from build123d import *

# Parameters (mm, degrees)
PAD_DEPTH       = 9
POCKET_DEPTH    = 6
SKETCH002_W     = 26.5
SKETCH002_H     = 35
POCKET001_DEPTH = 6
SKETCH003_W     = 192.75
SKETCH003_H     = 5.95
PAD001_DEPTH    = 3
SKETCH004_R     = 0.85
POCKET002_DEPTH = 541.411993
SKETCH005_W     = 26.5
SKETCH005_H     = 7.75
PAD002_DEPTH    = 3


with BuildPart() as part:
    # Sketch → Pad (new body)
    with BuildSketch(Plane.XY):
        with BuildLine():
            ThreePointArc((-92.5, 35), (-127.5, 0), (-92.5, -35))
            Line((-92.5, -35), (92.5, -35))
            ThreePointArc((92.5, -35), (127.5, 0), (92.5, 35))
            Line((-92.5, 35), (92.5, 35))
        make_face()
    extrude(amount=PAD_DEPTH)

    # Sketch001 (on Face6 of Pad) → Pocket (cut)
    with BuildSketch(Plane.XY.offset(9)):
        with BuildLine():
            ThreePointArc((-97.5, 6), (-103.5, 0), (-97.5, -6))
            Line((-97.5, -6), (97.5, -6))
            ThreePointArc((97.5, -6), (103.5, 0), (97.5, 6))
            Line((-97.5, 6), (97.5, 6))
        make_face()
    extrude(amount=-POCKET_DEPTH, mode=Mode.SUBTRACT)

    # Sketch002 (on Face5 of Pocket) → Pocket001 (cut)
    with BuildSketch(Plane.XY.offset(9)):
        with Locations((0, -17.5)):
            Rectangle(SKETCH002_W, SKETCH002_H)
    extrude(amount=-POCKET001_DEPTH, mode=Mode.SUBTRACT)

    # Sketch003 (on Face5 of Pocket001) → Pad001 (join)
    with BuildSketch(Plane.XY.offset(9)):
        with BuildLine():
            ThreePointArc((-92.5, 35), (-127.5, 0), (-92.5, -35))
            Line((-92.5, -35), (92.5, -35))
            ThreePointArc((92.5, -35), (127.5, 0), (92.5, 35))
            Line((-92.5, 35), (92.5, 35))
        make_face()
        Rectangle(SKETCH003_W, SKETCH003_H, mode=Mode.SUBTRACT)
    extrude(amount=PAD001_DEPTH)

    # Sketch004 (on Face12 of Pad001) → Pocket002 (cut, through all)
    with BuildSketch(Plane.XY.offset(12)):
        with Locations((-80, -8)):
            Circle(SKETCH004_R)
        with Locations((-63, -8)):
            Circle(SKETCH004_R)
        with Locations((-63, 8)):
            Circle(SKETCH004_R)
        with Locations((-80, 8)):
            Circle(SKETCH004_R)
    pocket002 = extrude(amount=-POCKET002_DEPTH, mode=Mode.SUBTRACT)

    # Sketch005 (on Face10 of Pocket002) → Pad002 (join)
    with BuildSketch(Plane.XY.offset(3)):
        with Locations((0, -37.125)):
            Rectangle(SKETCH005_W, SKETCH005_H)
    extrude(amount=PAD002_DEPTH)

    # Mirrored: Pocket002 across Sketch004 V_Axis
    add(pocket002.mirror(Plane(origin=(0, 0, 12), x_dir=(0, 0, 1), z_dir=(1, 0, 0))), mode=Mode.SUBTRACT)


solid = part.part
CAD build for the part. Positions are in the model's coordinates, mm. A direction names the side the tool comes from. Round coordinates to 2 decimals unless told otherwise and drop trailing zeros. Write each loop counter-clockwise with the first axis right and the second up, starting at its lowest first coordinate (ties: lowest second). Pieces come first, ordered by that corner, then holes. Notation, with made-up numbers: (65.5, -27) -> (107.5, -27) arc R35 ccw to (107.5, 8) -> close; hole circle Ø8 at (42.5, 30.5). An arc over 180 degrees is marked (long way). Answer as a JSON object with one key per item and string values.
(1) Band-saw the part on B-B, the plane y = -15. List the corners of the cut face in (x, z), then the cut area to 3 significant figures.
Reported:
{"outline": "(-124.12, 0) -> (124.12, 0) -> (124.12, 12) -> (-124.12, 12) -> close; hole (-13.25, 3) -> (13.25, 3) -> (13.25, 9) -> (-13.25, 9) -> close", "area": "2,820 mm^2"}
(2) Which spindle directions (+Z, -Z, +X, -X, +Y, -Y) get a long thin tool onto all of the face, cutting with end or side? Do faces 1 (the face through (-13.25, -21, 6)), 2 (the face through (0, -38, 3)), 3 (the face through (0, -37, 6)). Say none if no direction does.
Reported:
{"face 1": "none", "face 2": "-Z, +X, -X, -Y", "face 3": "-Y"}
(3) Pin check, flat tips, straight feed: P1, Ø1, axis at y = -32, z = 5, coming from the -X side; P2, Ø3.5, axis at y = -38, z = 4, coming from the +X side; P3, Ø4, axis at x = 91.5, z = 6, coming from the -Y side. Stop position of each tip, or through.
Reported:
{"P1": "stops at x = -107.76", "P2": "stops at x = 13.25", "P3": "stops at y = -35"}
(4) Band-saw the part on D-D, the plane y = 21.5. List the corners of the cut face in (x, z).
Reported:
{"outline": "(-120.12, 0) -> (120.12, 0) -> (120.12, 12) -> (-120.12, 12) -> close"}
(5) Probe probe 1 along Y at (x, z) = (-63, 3.5); probe 2 along Y at (x, z) = (63, 2.5); probe 3 along Y at (x, z) = (52, 4.5). List the from-to ranges inside material, lowest first. Write a range as [from, to].
Reported:
{"probe 1": "y = [-35, -8.85], [-7.15, -6], [6, 7.15], [8.85, 35]", "probe 2": "y = [-35, -8.85], [-7.15, 7.15], [8.85, 35]", "probe 3": "y = [-35, -6], [6, 35]"}
(6) Band-saw the part on C-C, the plane y = -31. List the corners of the cut face in (x, z).
Reported:
{"outline": "(-108.75, 0) -> (108.75, 0) -> (108.75, 12) -> (-108.75, 12) -> close; hole (-13.25, 3) -> (13.25, 3) -> (13.25, 9) -> (-13.25, 9) -> close"}
(7) Band-saw the part on A-A, the plane x = -20.5. List the corners of the cut face in (y, z) (3 decimals), then the cut area to 3 significant figures.
Reported:
{"outline": "(-35, 0) -> (35, 0) -> (35, 12) -> (2.975, 12) -> (2.975, 9) -> (6, 9) -> (6, 3) -> (-6, 3) -> (-6, 9) -> (-2.975, 9) -> (-2.975, 12) -> (-35, 12) -> close", "area": "750 mm^2"}
(8) Two-plate mould, pull along Y, no slides. Class faces 4 (the face through (13.25, -21, 6)), 5 (the face through (-127.49, 0.77, 5.92)), 6 (the face through (-2, 8, 12)), 7 (the face through (-1, 35, 6)): +Y half, -Y half, draft (parallel to the pull), parting line (faces both ways), or undercut.
Reported:
{"face 4": "undercut", "face 5": "parting line", "face 6": "draft", "face 7": "+Y half"}
